Part model, mm, in its own coordinate system. Face numbers are marked on the shaded views. A direction names the side the tool comes from. Give positions to 0.01 mm unless a question says otherwise; leave off trailing zeros. Write each loop counter-clockwise with the first axis right and the second up, starting at its lowest first coordinate (ties: lowest second). Pieces come first, ordered by that corner, then holes.
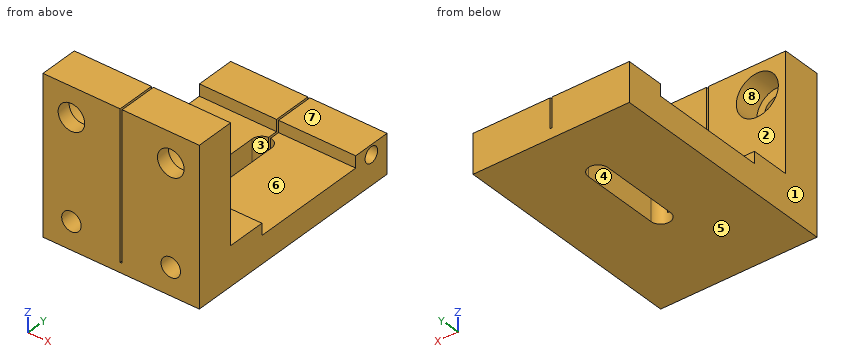
```python
from build123d import *

# Parameters (mm, degrees)
SKETCH1_W           = 40
SKETCH1_H           = 60
BOSS_EXTRUDE1_DEPTH = 10
CUT_EXTRUDE1_DEPTH  = 11
SKETCH5_W           = 3
SKETCH5_H           = 30
CUT_EXTRUDE4_DEPTH  = 41
SKETCH6_W           = 40
SKETCH6_H           = 10
BOSS_EXTRUDE2_DEPTH = 30
SKETCH8_W           = 0.5
SKETCH8_H           = 37.5
CUT_EXTRUDE7_DEPTH  = 60
SKETCH10_R          = 2
CUT_EXTRUDE10_DEPTH = 30
SKETCH12_R          = 3.4
SKETCH12_R_2        = 2.49
CUT_EXTRUDE13_DEPTH = 10
SKETCH14_R          = 5.375
CUT_EXTRUDE14_DEPTH = 6.5


with BuildPart() as part:
    # Sketch1 → Boss-Extrude1 (new body)
    with BuildSketch(Plane.XY):
        with Locations((-20, -30)):
            Rectangle(SKETCH1_W, SKETCH1_H)
    extrude(amount=BOSS_EXTRUDE1_DEPTH)

    # Sketch2 → Cut-Extrude1 (cut, through all)
    with BuildSketch(Plane.XY.offset(10)):
        with BuildLine():
            Line((-17.5, -15), (-17.5, -35))
            ThreePointArc((-17.5, -35), (-20, -37.5), (-22.5, -35))
            Line((-22.5, -35), (-22.5, -15))
            ThreePointArc((-22.5, -15), (-20, -12.5), (-17.5, -15))
        make_face()
    extrude(amount=-CUT_EXTRUDE1_DEPTH, mode=Mode.SUBTRACT)

    # Sketch5 → Cut-Extrude4 (cut, through all)
    with BuildSketch(Plane(origin=(0, 0, 0), x_dir=(0, 0, -1), z_dir=(1, 0, 0))):
        with Locations((-8.5, -25)):
            Rectangle(SKETCH5_W, SKETCH5_H)
    extrude(amount=-CUT_EXTRUDE4_DEPTH, mode=Mode.SUBTRACT)

    # Sketch6 → Boss-Extrude2 (add)
    with BuildSketch(Plane.XY.offset(10)):
        with Locations((-20, -55)):
            Rectangle(SKETCH6_W, SKETCH6_H)
    extrude(amount=BOSS_EXTRUDE2_DEPTH)

    # Sketch8 → Cut-Extrude7 (cut)
    with BuildSketch(Plane(origin=(0, 0, 0), x_dir=(1, 0, 0), z_dir=(0, 1, 0))):
        with Locations((-20, -21.25)):
            Rectangle(SKETCH8_W, SKETCH8_H)
    extrude(amount=-CUT_EXTRUDE7_DEPTH, mode=Mode.SUBTRACT)

    # Sketch10 → Cut-Extrude10 (cut)
    with BuildSketch(Plane(origin=(0, 0, 0), x_dir=(0, 0, -1), z_dir=(1, 0, 0))):
        with Locations((-7.5, -5)):
            Circle(SKETCH10_R)
    extrude(amount=-CUT_EXTRUDE10_DEPTH, mode=Mode.SUBTRACT)

    # Sketch12 → Cut-Extrude13 (cut)
    with BuildSketch(Plane.XZ.offset(60)):
        with Locations((-7.3, 32.43)):
            Circle(SKETCH12_R)
        with Locations((-32.73, 32.43)):
            Circle(SKETCH12_R)
        with Locations((-32.73, 7)):
            Circle(SKETCH12_R_2)
        with Locations((-7.3, 7)):
            Circle(SKETCH12_R_2)
    extrude(amount=-CUT_EXTRUDE13_DEPTH, mode=Mode.SUBTRACT)

    # Sketch14 → Cut-Extrude14 (cut)
    with BuildSketch(Plane(origin=(0, -50, 0), x_dir=(1, 0, 0), z_dir=(0, 1, 0))):
        with Locations((-32.73, -32.43)):
            Circle(SKETCH14_R)
        with Locations((-7.3, -32.43)):
            Circle(SKETCH14_R)
    extrude(amount=-CUT_EXTRUDE14_DEPTH, mode=Mode.SUBTRACT)


solid = part.part
```
1) Saw through at D-D, the plane x = -6. Write the cut outline in (y, z).
Answers follow:
outline: (-60, 0) - (0, 0) - (0, 10) - (-10, 10) - (-10, 7) - (-40, 7) - (-40, 10) - (-50, 10) - (-50, 27.21) - (-56.5, 27.21) - (-56.5, 29.29) - (-60, 29.29) - (-60, 9.12) - (-50, 9.12) - (-50, 4.88) - (-60, 4.88) - close; (-60, 35.57) - (-56.5, 35.57) - (-56.5, 37.65) - (-50, 37.65) - (-50, 40) - (-60, 40) - close; hole circle Ø4 at (-5, 7.5)
2) 3-axis set-ups, long thin cutter, end or side, ignore diameter. For the marked faces 4, 5, 6, 7 and 8: which of +Z, -Z, +X, -X, +Y, -Y reach the whole face in a straight line?
Answers follow:
face 4: +Z, -Z
face 5: -Z, +X, -X, +Y, -Y
face 6: +Z, +X, -X
face 7: +Z, +X, -X, +Y
face 8: +Y
3) Saw through at A-A, the plane y = -31. Write the cut outline in (x, z).
Answers follow:
outline: (-40, 0) - (-22.5, 0) - (-22.5, 7) - (-40, 7) - close; (-17.5, 0) - (0, 0) - (0, 7) - (-17.5, 7) - close
4) Two-plate mould, pull along Y, no slides. Class the marked faces 1, 2 and 3: +Y half, -Y half, draft (parallel to the pull), parting line (faces both ways), or undercut.
Answers follow:
face 1: draft
face 2: +Y half
face 3: undercut
5) Wall check: L1, parallel to Z at x = -7.3, y = -53.5 (3 decimals); L2, parallel to Y at x = -23, z = 7.5; L3, parallel to X at y = -52.5, z = 32.43 (3 decimals). Give the ranges that are in metal, low to high.
Answers follow:
L1: z = 0 to 4.51, 9.49 to 27.055, 37.805 to 40
L2: y = -60 to -40, -10 to -7, -3 to 0
L3: x = -40 to -38.105, -27.355 to -20.25, -19.75 to -12.675, -1.925 to 0
6) Pin check, flat tips, straight feed: pin 1 Ø8 at (x, y) = (-22, -20.5) entering from +Z; pin 2 Ø5 at (x, y) = (-8.5, -7) entering from +Z; pin 3 Ø7 at (y, z) = (-45, 29) entering from -X; pin 4 Ø3 at (x, z) = (-35, 30.5) entering from +Y. Stop position of each tip, or through.
Answers follow:
pin 1: stops at z = 7
pin 2: stops at z = 10
pin 3: passes through
pin 4: stops at y = -56.5
7) Saw through at C-C, the plane y = -54. Write the cut outline in (x, z) (3 decimals), then the cut area to 3 significant figures.
Answers follow:
outline: (-40, 0) - (0, 0) - (0, 40) - (-19.75, 40) - (-19.75, 2.5) - (-20.25, 2.5) - (-20.25, 40) - (-40, 40) - close; hole circle Ø10.75 at (-32.73, 32.43); hole circle Ø4.98 at (-32.73, 7); hole circle Ø10.75 at (-7.3, 32.43); hole circle Ø4.98 at (-7.3, 7)
area: 1,360 mm2
8) Saw through at B-B, the plane x = -32.73. Write the cut outline in (y, z) (3 decimals).
Answers follow:
outline: (-60, 0) - (0, 0) - (0, 10) - (-10, 10) - (-10, 7) - (-40, 7) - (-40, 10) - (-50, 10) - (-50, 27.055) - (-56.5, 27.055) - (-56.5, 29.03) - (-60, 29.03) - (-60, 9.49) - (-50, 9.49) - (-50, 4.51) - (-60, 4.51) - close; (-60, 35.83) - (-56.5, 35.83) - (-56.5, 37.805) - (-50, 37.805) - (-50, 40) - (-60, 40) - close
